Answer from the drawing. Dimensions are ordinates in mm from the lowest x, y and z of the part. A direction names the side the tool comes from. Give positions to 0.01 mm unless a question says otherwise; leave off trailing zeros. Order: outer loops, then holes, each group sorted by start corner. A loop starts at its lowest first (then second) coordinate and runs counter-clockwise, first axis right, second up.
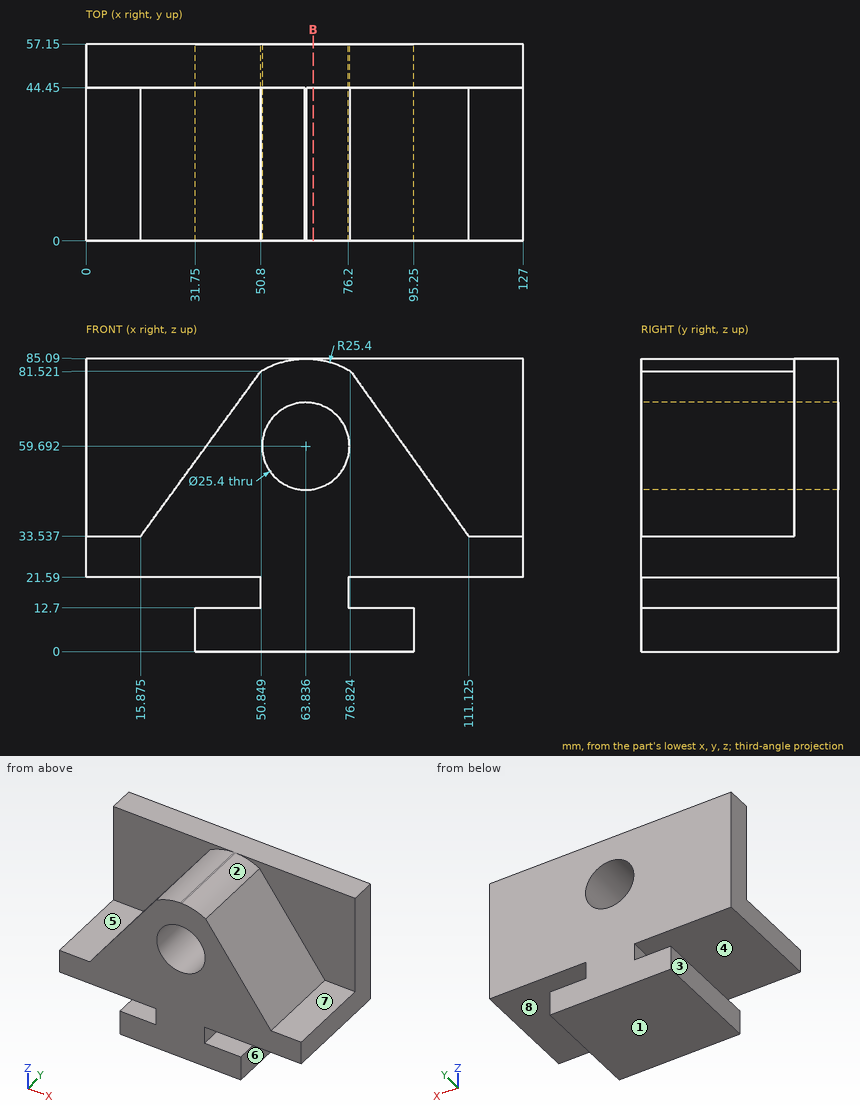
1) Given pin 1 (7 mm diameter, centred on y = 20.5, z = 15.5, fed in from +X); pin 2 (5.5 mm diameter, centred on x = 38.5, y = 20.5, fed in from +Z); pin 3 (2 mm diameter, centred on x = 13, z = 36, fed in from -Y), each flat-ended and moving along its own axis, determine where each tip first touches the part or whether it passes through.
Final values:
pin 1: stops at x = 95.25
pin 2: stops at z = 68.35
pin 3: stops at y = 44.45
2) For a pull along Z with two mould halves and no side action, classify the marked faces 1, 2, 3 and 4 as released by +Z, released by -Z, zero draft, split by the parting line, or undercut.
Final values:
face 1: released by -Z
face 2: released by +Z
face 3: zero draft
face 4: undercut
3) A tool of negligible diameter and unlimited length cuts with its end or side. For the marked faces 5, 6, 7 and 8, from which of +Z, -Z, +X, -X, +Y, -Y can it reach the whole face along a straight path? Write none if from no direction.
Final values:
face 5: +Z, -X, -Y
face 6: -Z, +X, +Y, -Y
face 7: +Z, +X, -Y
face 8: +X, +Y, -Y
4) Consider L1, parallel to Z at x = 33, y = 49.5; L2, parallel to Z at x = 31, y = 44.5; L3, parallel to Y at x = 12.5, z = 73.5. Determine where each line is inside the solid, lowest interval first.
Final values:
L1: z = 0 to 12.7, 21.59 to 85.09
L2: z = 21.59 to 85.09
L3: y = 44.45 to 57.15
5) The part is cut by section B-B on x = 66. Determine the outline of the cut face in (y, z).
Final values:
outline: (0, 0) - (57.15, 0) - (57.15, 47.18) - (0, 47.18) - close; (0, 72.21) - (57.15, 72.21) - (57.15, 85.09) - (44.45, 85.09) - (44.45, 85) - (0, 85) - close
